Here's how the part is built. I have some questions about the finished solid (model axes, mm). A direction names the side the tool comes from. Give positions to 0.01 mm unless a question says otherwise; leave off trailing zeros. Loops run counter-clockwise (first coordinate to the right, second up) from the corner with the lowest first, then second, coordinate; pieces in that order, holes last. Notation, with made-up numbers: (86, -24.5) - (114, -24.5) arc R17 ccw to (114, -9.5) - close; hole circle Ø2 at (-7, -4). An arc over 180 degrees is marked (long way). Return JSON: item names as keys, results as strings. Group by question number.
(1) If we section it at A-A (x = 492): Please give me the cut outline in (y, z), then the cut area to 3 significant figures.
(2) On a 3-axis mill with a long thin cutter (end or side, diameter ignored), from which of +Z, -Z, +X, -X, +Y, -Y can I reach the whole of each face in a straight line? I mean faces 4 (the flat face through (0, -197, -390)), 5 (the flat face through (199, -197, -36)). Say none if no direction works.
(3) If we section it at B-B (z = -237): Please give me the cut outline in (x, y), then the cut area to 3 significant figures.
(4) If we section it at C-C (y = -196): State how many separate pieces and enclosed holes the cut face has, then the cut area to 3 significant figures.
(5) I need wall thicknesses on probe 1 along X at (y, z) = (-145, -67.5); probe 2 along Z at (x, y) = (470.5, -28). Which ranges of each line are inside material? Lowest first, please. Write a range as [from, to].
(6) If we mould it in two halves opening along X, with no side actions, what happens to faces 1 (the flat face through (746, 0, -383)), 2 (the flat face through (1134, -197, -571)), 3 (the flat face through (1500, -197, -390))? For each: released by +X, released by -X, zero draft, split by the parting line, or undercut.
(7) For P1, Ø12, axis at x = 450, y = -304, coming from the +Z side, with a flat end and sliding along its axis, tell me the tip position at first contact or that it passes through.
```python
from build123d import *

# Parameters (mm, degrees)
F0_W     = 1500
F0_H     = 770
F0_W_2   = 330
F0_H_2   = 330
F1_DEPTH = 400


with BuildPart() as f1:
    # F0 (on Front) → F1 (new body)
    with BuildSketch(Plane.XZ):
        with Locations((750, -385)):
            Rectangle(F0_W, F0_H)
        with Locations((201, -569)):
            Rectangle(F0_W_2, F0_H_2, mode=Mode.SUBTRACT)
        with Locations((567, -569)):
            Rectangle(F0_W_2, F0_H_2, mode=Mode.SUBTRACT)
        with Locations((933, -569)):
            Rectangle(F0_W_2, F0_H_2, mode=Mode.SUBTRACT)
        with Locations((1299, -569)):
            Rectangle(F0_W_2, F0_H_2, mode=Mode.SUBTRACT)
        with Locations((201, -201)):
            Rectangle(F0_W_2, F0_H_2, mode=Mode.SUBTRACT)
        with Locations((567, -201)):
            Rectangle(F0_W_2, F0_H_2, mode=Mode.SUBTRACT)
        with Locations((933, -201)):
            Rectangle(F0_W_2, F0_H_2, mode=Mode.SUBTRACT)
        with Locations((1299, -201)):
            Rectangle(F0_W_2, F0_H_2, mode=Mode.SUBTRACT)
    extrude(amount=F1_DEPTH)


solid = f1.part
```
Values:
{
 "1": {"outline": "(-400, -770) - (0, -770) - (0, -734) - (-400, -734) - close; (-400, -404) - (0, -404) - (0, -366) - (-400, -366) - close; (-400, -36) - (0, -36) - (0, 0) - (-400, 0) - close", "area": "44,000 mm2"},
 "2": {"face 4": "+Z, -Z, -X, +Y, -Y", "face 5": "+Y, -Y"},
 "3": {"outline": "(0, -400) - (36, -400) - (36, 0) - (0, 0) - close; (366, -400) - (402, -400) - (402, 0) - (366, 0) - close; (732, -400) - (768, -400) - (768, 0) - (732, 0) - close; (1098, -400) - (1134, -400) - (1134, 0) - (1098, 0) - close; (1464, -400) - (1500, -400) - (1500, 0) - (1464, 0) - close", "area": "72,000 mm2"},
 "4": {"separate pieces": "1", "enclosed holes": "8", "area": "284,000 mm2"},
 "5": {"probe 1": "[0, 36], [366, 402], [732, 768], [1098, 1134], [1464, 1500]", "probe 2": "[-770, -734], [-404, -366], [-36, 0]"},
 "6": {"face 1": "zero draft", "face 2": "undercut", "face 3": "released by +X"},
 "7": {"P1": "z = 0"}
}
